from build123d import *

# Parameters (mm, degrees)
CROQUIS3_R              = 50
SALIENTE_EXTRUIR2_DEPTH = 10
CROQUIS4_R              = 5
SALIENTE_EXTRUIR3_DEPTH = 12
MATRIZC1_COUNT          = 12


with BuildPart() as part:
    # Croquis3 → Saliente-Extruir2 (new body)
    with BuildSketch(Plane(origin=(0, 0, 0), x_dir=(1, 0, 0), z_dir=(0, 1, 0))):
        with Locations(Location((0, 0, 0), (0, 0, 270))):
            Circle(CROQUIS3_R)
    extrude(amount=SALIENTE_EXTRUIR2_DEPTH)

    # Croquis4 → Saliente-Extruir3 (add)
    with BuildSketch(Plane(origin=(0, 10, 0), x_dir=(1, 0, 0), z_dir=(0, 1, 0))):
        with Locations(Location((0, 43.264151253, 0), (0, 0, 270))):
            Circle(CROQUIS4_R)
    saliente_extruir3 = extrude(amount=SALIENTE_EXTRUIR3_DEPTH)

    # MatrizC1: Saliente-Extruir3 ×12 about axis
    matrizc1_axis = Axis((0, 0, 0), (0, 1, 0))
    for i in range(1, MATRIZC1_COUNT):
        add(saliente_extruir3.rotate(matrizc1_axis, i * 360 / MATRIZC1_COUNT))


solid = part.part
For this review, take the finished solid that the model builds, in its own axes (mm). A direction names the side the tool comes from. Give positions to 0.01 mm unless a question says otherwise; leave off trailing zeros. Order: outer loops, then holes, each group sorted by start corner. A loop starts at its lowest first (then second) coordinate and runs counter-clockwise, first axis right, second up. Notation, with made-up numbers: (81.5, -37.75) -> (87.5, -37.75) arc R22 cw to (87.5, -15.75) -> close; hole circle Ø1 at (29, -14.75). An arc over 180 degrees is marked (long way). Write item = value, one per line.
1) We need section B-B, the plane y = 12.25. Count the separate pieces of the cut face and the enclosed holes in it, and give its area (3 significant figures).
Findings:
separate_pieces = 12
enclosed_holes = 0
area = 942 mm^2
2) Insertion check: pin 1 (10 mm diameter, centred on y = 10, z = -5.5, fed in from +X); pin 2 (3 mm diameter, centred on x = 29.5, z = 17, fed in from +Y); pin 3 (10 mm diameter, centred on x = 25, y = 6, fed in from +Z). Each pin has a flat end and moves straight along its axis. Give the tip position at first contact, or say it passes through.
Findings:
pin_1 = 50
pin_2 = 10
pin_3 = 45.83
3) We need section A-A, the plane x = 0. Give the boundary of the cut face in (y, z), and give its area (3 significant figures).
Findings:
outline = (0, -50) -> (10, -50) -> (10, -48.26) -> (22, -48.26) -> (22, -38.26) -> (10, -38.26) -> (10, 38.26) -> (22, 38.26) -> (22, 48.26) -> (10, 48.26) -> (10, 50) -> (0, 50) -> close
area = 1,240 mm^2
4) For faces 1 (the face through (0.22, 15.92, -48.26)), 2 (the face through (0, 22, -43)), list the 3-axis set-ups (+Z, -Z, +X, -X, +Y, -Y) from which the entire face can be reached by the end or side of a thin tool; tool diameter is ignored.
Findings:
face_1 = +Y
face_2 = +Z, -Z, +X, -X, +Y
5) We need section C-C, the plane z = 0. Give the boundary of the cut face in (x, y), and give its area (3 significant figures).
Findings:
outline = (-50, 0) -> (50, 0) -> (50, 10) -> (48.26, 10) -> (48.26, 22) -> (38.26, 22) -> (38.26, 10) -> (-38.26, 10) -> (-38.26, 22) -> (-48.26, 22) -> (-48.26, 10) -> (-50, 10) -> close
area = 1,240 mm^2
6) We need section D-D, the plane z = -40. Give the boundary of the cut face in (x, y).
Findings:
outline = (-30, 0) -> (30, 0) -> (30, 10) -> (25.94, 10) -> (25.94, 22) -> (17.32, 22) -> (17.32, 10) -> (3.79, 10) -> (3.79, 22) -> (-3.79, 22) -> (-3.79, 10) -> (-17.32, 10) -> (-17.32, 22) -> (-25.94, 22) -> (-25.94, 10) -> (-30, 10) -> close
7) To check wall thickness, follow L1, parallel to X at y = 21, z = -37; L2, parallel to Y at x = -9, z = -18; L3, parallel to X at y = 14, z = -1.5. State the ranges of each line that lie inside material, in increasing order. Write a range as from..to.
Findings:
L1 = -26.61..-16.65, 16.65..26.61
L2 = 0..10
L3 = -48.03..-38.49, 38.49..48.03
8) Draft analysis for pull direction Z (two halves, no side actions). For faces 3 (the face through (15.02, 4.93, 47.69)), 4 (the face through (-22, 22, -38)), 5 (the face through (38.97, 15.92, 26.4)), state which applies: pulls with the +Z half, pulls with the -Z half, needs draft (parallel to the pull), parting line crosses it, or undercut.
Findings:
face_3 = parting line crosses it
face_4 = needs draft
face_5 = undercut
